Could you check a few things on this model? Use its own coordinates, in mm. Face numbers are marked on the shaded views. Give positions to 0.01 mm unless a question says otherwise; leave off trailing zeros. Loops run counter-clockwise (first coordinate to the right, second up) from the corner with the lowest first, then second, coordinate; pieces in that order, holes last.
1. I need wall thicknesses on line 1 along Y through (x, z) = (0, 10); line 2 along X through (y, z) = (-2, 4.5); line 3 along X through (y, z) = (-3.5, 8). Which ranges of each line are inside material? Lowest first, please.
2. Imagine slicing it at A-A (y = 0). List the corners of the cut face in (x, z) for me.
3. For P1, Ø1.5, axis at y = -3.5, z = 8, coming from the +X side; P2, Ø3, axis at y = -2.5, z = 7.5, coming from the -X side, each with a flat end and sliding along its axis, tell me the tip position at first contact or that it passes through.
4. Imagine slicing it at C-C (z = 10.75). List the corners of the cut face in (x, y) for me, plus the area to 3 significant figures.
5. Thinking about a two-plate mould opening in Y: for the marked faces 1, 2 and 3, which applies, +Y half, -Y half, draft (parallel to the pull), parting line (faces both ways), or undercut?
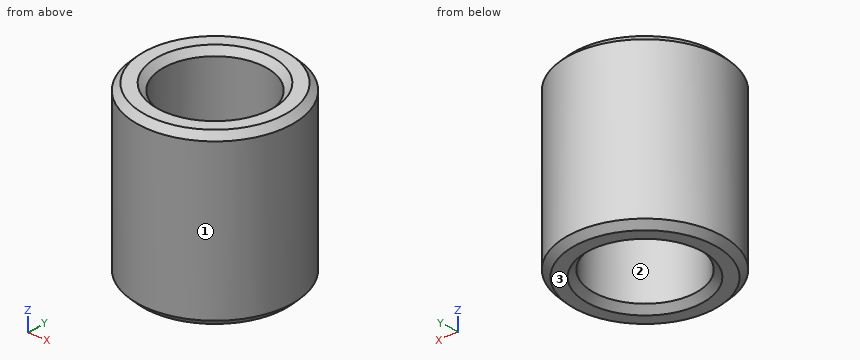
```python
from build123d import *

# Parameters (mm, degrees)
F0_R     = 6
F0_R_2   = 4
F1_DEPTH = 13
F2_SIZE  = 0.5
F3_SIZE  = 0.5
F4_SIZE  = 0.5


with BuildPart() as f1:
    # F0 (on Top) → F1 (new body)
    with BuildSketch(Plane.XY):
        Circle(F0_R)
        Circle(F0_R_2, mode=Mode.SUBTRACT)
    extrude(amount=F1_DEPTH)

    # F2
    f2_edges = [f1.edges().sort_by_distance(p)[0] for p in [
        (-4, 0, 13),
    ]]
    chamfer(f2_edges, length=F2_SIZE)

    # F3
    f3_edges = [f1.edges().sort_by_distance(p)[0] for p in [
        (-4, 0, 0),
    ]]
    chamfer(f3_edges, length=F3_SIZE)

    # F4
    f4_edges = [f1.edges().sort_by_distance(p)[0] for p in [
        (-6, 0, 0),
        (-6, 0, 13),
    ]]
    chamfer(f4_edges, length=F4_SIZE)


solid = f1.part
```
Derived:
1. line 1: y = -6 to -4, 4 to 6
1. line 2: x = -5.66 to -3.46, 3.46 to 5.66
1. line 3: x = -4.87 to -1.94, 1.94 to 4.87
2. outline: (-6, 0.5) - (-5.5, 0) - (-4.5, 0) - (-4, 0.5) - (-4, 12.5) - (-4.5, 13) - (-5.5, 13) - (-6, 12.5) - close; (4, 0.5) - (4.5, 0) - (5.5, 0) - (6, 0.5) - (6, 12.5) - (5.5, 13) - (4.5, 13) - (4, 12.5) - close
3. P1: stops at x = 5.33
3. P2: stops at x = -5.92
4. outline: circle Ø12 at (0, 0); hole circle Ø8 at (0, 0)
4. area: 62.8 mm2
5. face 1: parting line
5. face 2: undercut
5. face 3: draft
